Design review of the part built by this model. Coordinates are the model's own, in mm. Face numbers are marked on the shaded views. A direction names the side the tool comes from. Coordinates: 2 decimals unless noted, no trailing zeros. Order: outer loops, then holes, each group sorted by start corner. A loop starts at its lowest first (then second) coordinate and runs counter-clockwise, first axis right, second up. Notation, with made-up numbers: M 12.5,-5 L 42.5,-5 A23 ccw 42.5,11 Z; hole C -26.75,-19 d1. An arc over 180 degrees is marked long. Answer as a JSON object with one key per item and string values.
from build123d import *

# Parameters (mm, degrees)
ESQUISSE1_W             = 30
ESQUISSE1_H             = 20
BOSS_EXTRU_1_DEPTH      = 2
ESQUISSE2_R             = 0.75
ENL_V_MAT_EXTRU_1_DEPTH = 2
ESQUISSE3_R             = 1.25
BOSS_EXTRU_2_DEPTH      = 2
ESQUISSE4_W             = 5.380750915
ESQUISSE4_H             = 5.957728466
BOSS_EXTRU_3_DEPTH      = 5


with BuildPart() as part:
    # Esquisse1 → Boss.-Extru.1 (new body)
    with BuildSketch(Plane(origin=(0, 0, 0), x_dir=(1, 0, 0), z_dir=(0, 1, 0))):
        Rectangle(ESQUISSE1_W, ESQUISSE1_H)
    extrude(amount=BOSS_EXTRU_1_DEPTH)

    # Esquisse2 → Enlèv. mat.-Extru.1 (cut)
    with BuildSketch(Plane(origin=(0, 2, 0), x_dir=(1, 0, 0), z_dir=(0, 1, 0))):
        with Locations(Location((-13.777247076, -8.688354012, 0), (0, 0, 270))):
            Circle(ESQUISSE2_R)
    enl_v_mat_extru_1 = extrude(amount=-ENL_V_MAT_EXTRU_1_DEPTH, mode=Mode.SUBTRACT)

    # Symétrie1: Enlèv. mat.-Extru.1 across plane
    add(enl_v_mat_extru_1.mirror(Plane.XY), mode=Mode.SUBTRACT)

    # Esquisse3 → Boss.-Extru.2 (add)
    with BuildSketch(Plane(origin=(0, 2, 0), x_dir=(1, 0, 0), z_dir=(0, 1, 0))):
        with Locations(Location((-4.31314717, 0.651626551, 0), (0, 0, 270))):
            Circle(ESQUISSE3_R)
    extrude(amount=BOSS_EXTRU_2_DEPTH)

    # Esquisse4 → Boss.-Extru.3 (add)
    with BuildSketch(Plane(origin=(0, 2, 0), x_dir=(1, 0, 0), z_dir=(0, 1, 0))):
        with Locations((12.309624542, 0.744716058)):
            Rectangle(ESQUISSE4_W, ESQUISSE4_H)
    extrude(amount=BOSS_EXTRU_3_DEPTH)


solid = part.part
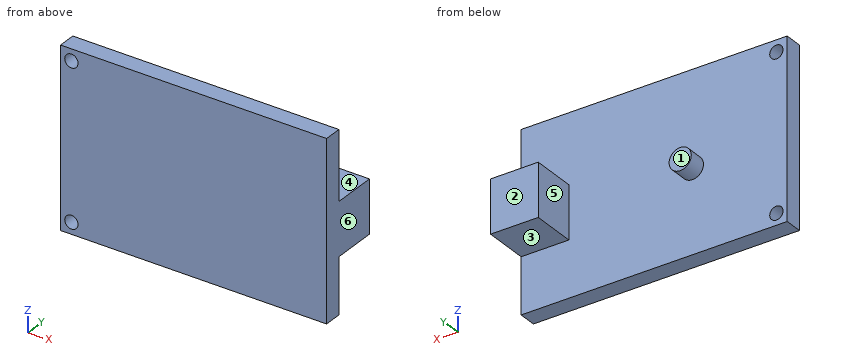
1) To check wall thickness, follow L1, parallel to Y at x = -8, z = 2.25; L2, parallel to X at y = 6.5, z = -1.25; L3, parallel to Z at x = 9.75, y = 6. State the ranges of each line that lie inside material, in increasing order.
Taken from the geometry:
{"L1": "y = 0 to 2", "L2": "x = 9.62 to 15", "L3": "z = -3.72 to 2.23"}
2) Insertion check: pin 1 Ø4 at (y, z) = (5, -2) entering from -X; pin 2 Ø3 at (x, z) = (-4.5, -0.5) entering from +Y. Each pin has a flat end and moves straight along its axis. Give the tip position at first contact, or say it passes through.
Taken from the geometry:
{"pin 1": "stops at x = -5.56", "pin 2": "stops at y = 4"}
3) Add section D-D (y = 5.75). State the section outline as (x, z) points.
Taken from the geometry:
{"outline": "M 9.62,-3.72 L 15,-3.72 L 15,2.23 L 9.62,2.23 Z"}
4) Tool access review of the marked faces 1, 2 and 3: name each direction out of +Z, -Z, +X, -X, +Y, -Y from which nothing blocks a thin tool from reaching the whole face with its end or side.
Taken from the geometry:
{"face 1": "+Z, -Z, -X, +Y", "face 2": "+Z, -Z, +X, -X, +Y", "face 3": "-Z, +X, -X, +Y"}
5) Mouldability with a two-part tool opening along X and no side actions: class the marked faces 4, 5 and 6 as released by +X, released by -X, zero draft, split by the parting line, or undercut.
Taken from the geometry:
{"face 4": "zero draft", "face 5": "undercut", "face 6": "released by +X"}
6) Add section B-B (y = 2.75). State the section outline as (x, z) points, and give its area (3 significant figures).
Taken from the geometry:
{"outline": "C -4.31,-0.65 d2.5; M 9.62,-3.72 L 15,-3.72 L 15,2.23 L 9.62,2.23 Z", "area": "37.0 mm2"}
7) Add section C-C (z = 1.25). State the section outline as (x, y) points, and give its area (3 significant figures).
Taken from the geometry:
{"outline": "M -15,0 L 15,0 L 15,7 L 9.62,7 L 9.62,2 L -15,2 Z", "area": "86.9 mm2"}
8) Add section A-A (x = 12.75). State the section outline as (y, z) points, and give its area (3 significant figures).
Taken from the geometry:
{"outline": "M 0,-10 L 2,-10 L 2,-3.72 L 7,-3.72 L 7,2.23 L 2,2.23 L 2,10 L 0,10 Z", "area": "69.8 mm2"}
